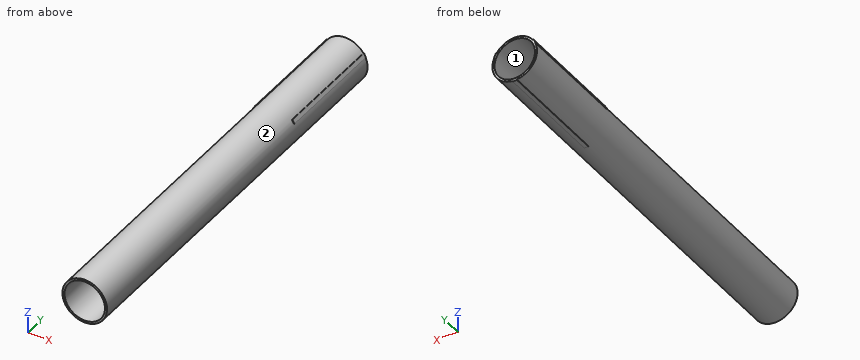
```python
from build123d import *

# Parameters (mm, degrees)
ESBO_O1_R                = 21.5
ESBO_O1_R_2              = 19.5
RESSALTO_EXTRUS_O1_DEPTH = 400
RESSALTO_EXTRUS_O3_DEPTH = 110
PADR_OCIRCULAR2_COUNT    = 3


with BuildPart() as part:
    # Esboço1 → Ressalto-extrusão1 (new body)
    with BuildSketch(Plane(origin=(0, 0, 0), x_dir=(1, 0, 0), z_dir=(0, 1, 0))):
        with Locations(Location((0, 0, 0), (0, 0, 270))):
            Circle(ESBO_O1_R)
        with Locations(Location((0, 0, 0), (0, 0, 270))):
            Circle(ESBO_O1_R_2, mode=Mode.SUBTRACT)
    extrude(amount=RESSALTO_EXTRUS_O1_DEPTH)

    # Esboço2 → Ressalto-extrusão3 (add)
    with BuildSketch(Plane(origin=(0, 400, 0), x_dir=(1, 0, 0), z_dir=(0, 1, 0))):
        Polygon((2, 21.930506272), (2, 21.234864033), (0, 21.5), (-1.998917515, 21.234864033), (-1.998917515, 21.930506272), align=None)
    ressalto_extrus_o3 = extrude(amount=-RESSALTO_EXTRUS_O3_DEPTH)

    # PadrãoCircular2: Ressalto-extrusão3 ×3 about axis
    padr_ocircular2_axis = Axis((0, 0, 0), (0, 1, 0))
    for i in range(1, PADR_OCIRCULAR2_COUNT):
        add(ressalto_extrus_o3.rotate(padr_ocircular2_axis, i * 360 / PADR_OCIRCULAR2_COUNT))


solid = part.part
```
Geometry check sheet. Reference: the model listing, model coordinates, mm. Face numbers are marked on the shaded views. A direction names the side the tool comes from. Round coordinates to 2 decimals unless told otherwise and drop trailing zeros. Order: outer loops, then holes, each group sorted by start corner. A loop starts at its lowest first (then second) coordinate and runs counter-clockwise, first axis right, second up. Notation, with made-up numbers: (-1.75, -25) - (11.25, -25) arc R17 cw to (11.25, -11) - close; hole circle Ø2 at (-1.5, -37.5). An arc over 180 degrees is marked (long way). Use a Markdown table: item, result. Add a question column.
1) Gauge pin test, flat ends, axial feed: P1, Ø2, axis at y = 44, z = -10.5, coming from the -X side; P2, Ø1.5, axis at y = 355, z = 4, coming from the -X side; P3, Ø0.7, axis at x = 19, z = 11, coming from the -Y side. Record the tip position at first contact, or that the pin passes through.
2) Section check A-A (y = 309). Record the cut outline in (x, z), then the cut area to 3 significant figures.
3) Section check C-C (x = -13). Record the cut outline in (y, z), then the cut area to 3 significant figures.
4) Thickness scan on line 1 along X through (y, z) = (179.5, 1.5); line 2 along X through (y, z) = (48.5, 1); line 3 along Z through (x, y) = (1.5, 355). Record the ranges inside material, lowest first.
5) Set-up check for the marked faces 1 and 2: record each of +Z, -Z, +X, -X, +Y, -Y from which the full face is reachable in a straight line by a thin tool's end or side.
6) Section check D-D (y = 99.5). Record the cut outline in (x, z), then the cut area to 3 significant figures.
7) Section check B-B (z = 0). Record the cut outline in (x, y).
Established:
| question | item | result |
|---|---|---|
| 1 | P1 | x = -19.29 |
| 1 | P2 | x = -21.25 |
| 1 | P3 | y = 290 |
| 2 | outline | (-19.99, 9.23) - (-19.54, 8.97) arc R21.5 ccw to (-2, -21.41) - (-2, -21.93) - (2, -21.93) - (2, -21.41) arc R21.5 ccw to (19.54, 8.97) - (19.99, 9.23) - (17.99, 12.7) - (17.54, 12.44) arc R21.5 ccw to (-17.54, 12.43) - (-17.99, 12.7) - close; hole circle Ø39 at (0, 0) |
| 2 | area | 263 mm2 |
| 3 | outline | (0, -17.12) - (400, -17.12) - (400, -14.53) - (0, -14.53) - close; (0, 14.53) - (400, 14.53) - (400, 17.12) - (0, 17.12) - close |
| 3 | area | 2,070 mm2 |
| 4 | line 1 | -21.45 to -19.44, 19.44 to 21.45 |
| 4 | line 2 | -21.48 to -19.47, 19.47 to 21.48 |
| 4 | line 3 | -21.93 to -19.44, 19.44 to 21.45 |
| 5 | face 1 | +Y, -Y |
| 5 | face 2 | -Y |
| 6 | outline | circle Ø43 at (0, 0); hole circle Ø39 at (0, 0) |
| 6 | area | 258 mm2 |
| 7 | outline | (-21.5, 0) - (-19.5, 0) - (-19.5, 400) - (-21.5, 400) - close; (19.5, 0) - (21.5, 0) - (21.5, 400) - (19.5, 400) - close |
